The model under review builds one solid part; all positions refer to its coordinate system, in mm. A direction names the side the tool comes from. Round coordinates to 2 decimals unless told otherwise and drop trailing zeros. Order: outer loops, then holes, each group sorted by start corner. A loop starts at its lowest first (then second) coordinate and runs counter-clockwise, first axis right, second up.
from build123d import *

# Parameters (mm, degrees)
CYLINDER002_R     = 11.25
CYLINDER002_DEPTH = 14
CYLINDER001_R     = 7.5
CYLINDER001_DEPTH = 29
CYLINDER_R        = 27
CYLINDER_DEPTH    = 29


with BuildPart() as cylinder002:
    # Cylinder002 → Cylinder002 (new body)
    with BuildSketch(Plane.XY.offset(15)):
        Circle(CYLINDER002_R)
    extrude(amount=CYLINDER002_DEPTH)


with BuildPart() as fusion:
    # Cylinder001 → Cylinder001 (new body)
    with BuildSketch(Plane.XY):
        Circle(CYLINDER001_R)
    extrude(amount=CYLINDER001_DEPTH)

    # Fusion: union Cylinder002
    add(cylinder002.part)


with BuildPart() as singleadapter:
    # Cylinder → Cylinder (new body)
    with BuildSketch(Plane.XY):
        Circle(CYLINDER_R)
    extrude(amount=CYLINDER_DEPTH)

    # Cut: cut Fusion
    add(fusion.part, mode=Mode.SUBTRACT)


solid = singleadapter.part
(1) We need section A-A (y = 0). Give the boundary of the cut face in (x, z).
(2) We need section D-D (y = 9). Give the boundary of the cut face in (x, z).
(3) Tool access review of faces 4 (the flat face through (6, -6, 0)), 5 (the cylindrical face through (5.19, -9.98, 21.9)): name each direction out of +Z, -Z, +X, -X, +Y, -Y from which nothing blocks a thin tool from reaching the whole face with its end or side.
(4) The part is to be moulded in two halves that separate along Y. For faces 1 (the cylindrical face through (-5.85, -26.36, 14.3)), 2 (the flat face through (12, 0, 29)), 3 (the flat face through (7.3, -2.3, 15)), say which applies: pulls with the +Y half, pulls with the -Y half, needs draft (parallel to the pull), parting line crosses it, or undercut.
(5) Clearance check with flat-ended pins moving along their axes: P1, Ø1.5, axis at y = 15, z = 13, coming from the +X side; P2, Ø1, axis at y = -1.5, z = 25.5, coming from the +X side; P3, Ø10, axis at x = -18, y = 12.5, coming from the -Z side; P4, Ø4, axis at x = -15.5, z = 22.5, coming from the +Y side. State where each tip first meets the part, or that it passes through.
(6) To check wall thickness, follow L1, parallel to Y at x = 0, z = 10.5; L2, parallel to Y at x = 0, z = 23.25; L3, parallel to Z at x = -8, y = 5.5. State the ranges of each line that lie inside material, in increasing order.
(7) We need section C-C (z = 25.25). Give the boundary of the cut face in (x, y), and give its area (3 significant figures).
Verdict:
1. outline: (-27, 0) - (-7.5, 0) - (-7.5, 15) - (-11.25, 15) - (-11.25, 29) - (-27, 29) - close; (7.5, 0) - (27, 0) - (27, 29) - (11.25, 29) - (11.25, 15) - (7.5, 15) - close
2. outline: (-25.46, 0) - (25.46, 0) - (25.46, 29) - (6.75, 29) - (6.75, 15) - (-6.75, 15) - (-6.75, 29) - (-25.46, 29) - close
3. face 4: -Z, +X, -X, +Y, -Y
3. face 5: +Z
4. face 1: parting line crosses it
4. face 2: needs draft
4. face 3: undercut
5. P1: stops at x = 22.93
5. P2: stops at x = 26.98
5. P3: stops at z = 0
5. P4: stops at y = 23.38
6. L1: y = -27 to -7.5, 7.5 to 27
6. L2: y = -27 to -11.25, 11.25 to 27
6. L3: z = 0 to 15
7. outline: circle Ø54 at (0, 0); hole circle Ø22.5 at (0, 0)
7. area: 1,890 mm2
